Part model, mm, in its own coordinate system. Round coordinates to 2 decimals unless told otherwise and drop trailing zeros. Loops run counter-clockwise (first coordinate to the right, second up) from the corner with the lowest first, then second, coordinate; pieces in that order, holes last. Notation, with made-up numbers: (74, 86.25) -> (129, 86.25) arc R25 cw to (129, 100.25) -> close; hole circle Ø8 at (32, 49.25). An arc over 180 degrees is marked (long way). Answer as CSV lines item,"result".
from build123d import *

# Parameters (mm, degrees)
BOSS_EXTRUDE1_DEPTH = 12.7
SKETCH2_R           = 12.7
CUT_EXTRUDE1_DEPTH  = 203.2


with BuildPart() as part:
    # Sketch1 → Boss-Extrude1 (new body)
    with BuildSketch(Plane.XY):
        Polygon((0, 0), (0, 605), (260.366426726, 605), (1315, 400), (1315, 0), align=None)
    extrude(amount=BOSS_EXTRUDE1_DEPTH)

    # Sketch2 → Cut-Extrude1 (cut)
    with BuildSketch(Plane(origin=(0, 0, 0), x_dir=(-1, 0, 0), z_dir=(0, 0, -1))):
        with Locations((-1219.75, 203.2)):
            Circle(SKETCH2_R)
    extrude(amount=-CUT_EXTRUDE1_DEPTH, mode=Mode.SUBTRACT)


solid = part.part
Q1. Saw through at A-A, the plane y = 203.2. Write the cut outline in (x, z).
Geometry results:
outline,"(0, 0) -> (1207.05, 0) -> (1207.05, 12.7) -> (0, 12.7) -> close; (1232.45, 0) -> (1315, 0) -> (1315, 12.7) -> (1232.45, 12.7) -> close"
Q2. Saw through at B-B, the plane z = 2.5. Write the cut outline in (x, y), then the cut area to 3 significant figures.
Geometry results:
outline,"(0, 0) -> (1315, 0) -> (1315, 400) -> (260.37, 605) -> (0, 605) -> close; hole circle Ø25.4 at (1219.75, 203.2)"
area,"687,000 mm2"
Q3. Drop flat-ended pins along their axis: P1, Ø1.5, axis at x = 449.5, z = 1.5, coming from the +Y side; P2, Ø1, axis at x = 550.5, z = 2, coming from the +Y side; P3, Ø23, axis at x = 1219.75, y = 203.2, coming from the -Z side. Give the stop position or say it passes through.
Geometry results:
P1,"y = 568.38"
P2,"y = 548.7"
P3,"through"
Q4. Saw through at D-D, the plane x = 477. Write the cut outline in (y, z).
Geometry results:
outline,"(0, 0) -> (562.89, 0) -> (562.89, 12.7) -> (0, 12.7) -> close"
Q5. Drill centre lines: line 1 along Y through (x, z) = (1219.75, 7); line 2 along Y through (x, z) = (1180.5, 2.5); line 3 along Y through (x, z) = (277.5, 8). Where is each one in solid material? Low to high.
Geometry results:
line 1,"0 to 190.5, 215.9 to 418.51"
line 2,"0 to 426.14"
line 3,"0 to 601.67"
Q6. Saw through at C-C, the plane x = 1219.75. Write the cut outline in (y, z), then the cut area to 3 significant figures.
Geometry results:
outline,"(0, 0) -> (190.5, 0) -> (190.5, 12.7) -> (0, 12.7) -> close; (215.9, 0) -> (418.51, 0) -> (418.51, 12.7) -> (215.9, 12.7) -> close"
area,"4,990 mm2"
